Verification items for the finished model (mm, model axes). Give positions to 0.01 mm unless a question says otherwise; leave off trailing zeros. Order: outer loops, then holes, each group sorted by start corner. A loop starts at its lowest first (then second) coordinate and runs counter-clockwise, first axis right, second up. Notation, with made-up numbers: (-34, 10.5) -> (-1, 10.5) arc R31 cw to (-1, 36.5) -> close; hole circle Ø8 at (85, -7.5). An arc over 180 degrees is marked (long way). Return JSON: item names as keys, results as strings. Group by question number.
(1) Cross-section at C-C on y = 103.5. Enter the section's corners in (x, z), then the cut area to 3 significant figures.
(2) Cross-section at D-D on z = 1.6. State how many separate pieces and enclosed holes the cut face has, then the cut area to 3 significant figures.
(3) Cross-section at A-A on y = -97.5. Enter the section's corners in (x, z).
(4) Cross-section at B-B on x = 73. Enter the section's corners in (y, z).
(5) Thickness scan on line 1 along X through (y, z) = (-199, 3.45); line 2 along X through (y, z) = (43, 2.65); line 3 along Y through (x, z) = (-137, 1.25). Record the ranges inside material, lowest first.
(6) Depth check by flat-ended pin: pin 1 Ø2 at (y, z) = (-225.5, 2) entering from +X; pin 2 Ø1.5 at (x, z) = (79, 2.5) entering from -Y; pin 3 Ø1.3 at (y, z) = (-197.5, 1.5) entering from -X. Enter the tip coordinate at first touch or a pass-through.
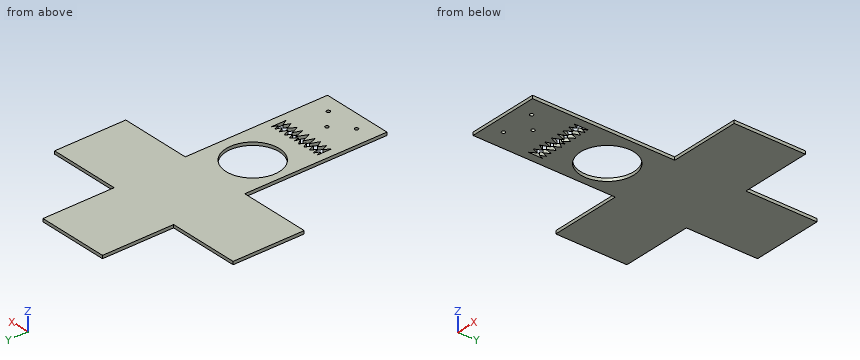
from build123d import *

# Parameters (mm, degrees)
F0_W     = 101.6
F0_H     = 101.6
F0_R     = 38.1
F0_R_2   = 2.5019
F1_DEPTH = 4.318
F2_DEPTH = 4.318


with BuildPart() as f1:
    # F0 (on Top) → F1 (new body)
    with BuildSketch(Plane.XY):
        with Locations((-104.021908, -24.545676)):
            Rectangle(F0_W, F0_H)
        with Locations((-2.421908, -24.545676)):
            Rectangle(F0_W, F0_H)
        with Locations((-2.421908, 77.054324)):
            Rectangle(F0_W, F0_H)
        with Locations((99.178092, -24.545676)):
            Rectangle(F0_W, F0_H)
        with Locations((-2.421908, -126.145676)):
            Rectangle(F0_W, F0_H)
        with Locations((-4.234652, -127.733991)):
            Circle(F0_R, mode=Mode.SUBTRACT)
        with Locations((-2.421908, -227.745676)):
            Rectangle(F0_W, F0_H)
        with Locations((-26.502896, -257.383049)):
            Circle(F0_R_2, mode=Mode.SUBTRACT)
        with Locations((21.65908, -257.383049)):
            Circle(F0_R_2, mode=Mode.SUBTRACT)
        with Locations((-2.421908, -235.197216)):
            Circle(F0_R_2, mode=Mode.SUBTRACT)
        Polygon((-41.561957, -209.521994), (-41.561957, -188.174039), (-38.587328, -195.748523), (-35.364017, -188.174039), (-32.320578, -196.259379), (-27.629388, -188.174039), (-24.196096, -197.991371), (-19.147361, -188.174039), (-14.316184, -195.874706), (-10.345475, -188.174039), (-3.992576, -195.874706), (-2.421908, -188.174039), (-0.85124, -195.874706), (5.501659, -188.174039), (9.472368, -195.874706), (14.303545, -188.174039), (19.35228, -197.991371), (22.785572, -188.174039), (27.476761, -196.259379), (30.520201, -188.174039), (33.743512, -195.748523), (36.718141, -188.174039), (36.718141, -209.521994), (31.677574, -200.754404), (27.82803, -209.521994), (23.414299, -199.966282), (17.148117, -209.521994), (12.626316, -198.055878), (8.395368, -209.521994), (3.620354, -195.874706), (-2.421908, -209.521994), (-8.464171, -195.874706), (-13.239184, -209.521994), (-17.470133, -198.055878), (-21.991933, -209.521994), (-28.258115, -199.966282), (-32.671846, -209.521994), (-36.52139, -200.754404), align=None, mode=Mode.SUBTRACT)
    extrude(amount=F1_DEPTH)

    # F0 (on Top) → F2 (join)
    with BuildSketch(Plane.XY):
        with Locations((-2.421908, 77.054324)):
            Rectangle(F0_W, F0_H)
        with Locations((-104.021908, -24.545676)):
            Rectangle(F0_W, F0_H)
        with Locations((99.178092, -24.545676)):
            Rectangle(F0_W, F0_H)
        with Locations((-2.421908, -126.145676)):
            Rectangle(F0_W, F0_H)
        with Locations((-4.234652, -127.733991)):
            Circle(F0_R, mode=Mode.SUBTRACT)
        with Locations((-2.421908, -227.745676)):
            Rectangle(F0_W, F0_H)
        with Locations((-26.502896, -257.383049)):
            Circle(F0_R_2, mode=Mode.SUBTRACT)
        with Locations((21.65908, -257.383049)):
            Circle(F0_R_2, mode=Mode.SUBTRACT)
        with Locations((-2.421908, -235.197216)):
            Circle(F0_R_2, mode=Mode.SUBTRACT)
        Polygon((-41.561957, -209.521994), (-41.561957, -188.174039), (-38.587328, -195.748523), (-35.364017, -188.174039), (-32.320578, -196.259379), (-27.629388, -188.174039), (-24.196096, -197.991371), (-19.147361, -188.174039), (-14.316184, -195.874706), (-10.345475, -188.174039), (-3.992576, -195.874706), (-2.421908, -188.174039), (-0.85124, -195.874706), (5.501659, -188.174039), (9.472368, -195.874706), (14.303545, -188.174039), (19.35228, -197.991371), (22.785572, -188.174039), (27.476761, -196.259379), (30.520201, -188.174039), (33.743512, -195.748523), (36.718141, -188.174039), (36.718141, -209.521994), (31.677574, -200.754404), (27.82803, -209.521994), (23.414299, -199.966282), (17.148117, -209.521994), (12.626316, -198.055878), (8.395368, -209.521994), (3.620354, -195.874706), (-2.421908, -209.521994), (-8.464171, -195.874706), (-13.239184, -209.521994), (-17.470133, -198.055878), (-21.991933, -209.521994), (-28.258115, -199.966282), (-32.671846, -209.521994), (-36.52139, -200.754404), align=None, mode=Mode.SUBTRACT)
    extrude(amount=F2_DEPTH)


solid = f1.part
Verdict:
{
 "1": {"outline": "(-53.22, 0) -> (48.38, 0) -> (48.38, 4.32) -> (-53.22, 4.32) -> close", "area": "439 mm²"},
 "2": {"separate pieces": "1", "enclosed holes": "5", "area": "56,400 mm²"},
 "3": {"outline": "(-53.22, 0) -> (-27.42, 0) -> (-27.42, 4.32) -> (-53.22, 4.32) -> close; (18.95, 0) -> (48.38, 0) -> (48.38, 4.32) -> (18.95, 4.32) -> close"},
 "4": {"outline": "(-75.35, 0) -> (26.25, 0) -> (26.25, 4.32) -> (-75.35, 4.32) -> close"},
 "5": {"line 1": "-53.22 to -41.56, -17.84 to -17.12, -9.56 to -7.08, 2.24 to 4.71, 12.28 to 13, 36.72 to 48.38", "line 2": "-53.22 to 48.38", "line 3": "-75.35 to 26.25"},
 "6": {"pin 1": "x = 48.38", "pin 2": "y = -75.35", "pin 3": "x = -53.22"}
}
